Input: dimensioned drawing with shaded views. Units: mm. Origin: part minimum x, y, z. A direction names the side the tool comes from. Round coordinates to 2 decimals unless told otherwise and drop trailing zeros. Write each loop counter-clockwise with the first axis right and the second up, starting at its lowest first coordinate (ties: lowest second). Pieces come first, ordered by that corner, then holes. Notation, with made-up numbers: M -13,34.25 L 37,34.25 A11 cw 37,53.25 Z; hole C 48,80.25 d2. An arc over 180 degrees is marked long. Answer in a Markdown table with one row per item. Add a question column.
Item 1: Material intervals for probe 1 along Y at (x, z) = (6.35, 1.75) (1 decimal); probe 2 along Z at (x, y) = (8, 80); probe 3 along Y at (x, z) = (6.25, 0.5), sorted ascending.
Item 2: Set-up query: the marked faces 1, 2 and 3. Return all of +Z, -Z, +X, -X, +Y, -Y with unobstructed straight access to the full face (end or side cutting, diameter ignored); none if empty.
Item 3: Cut plane A-A on x = 6.35. Give the number of separate pieces and of enclosed holes in the cut face, and give its area (3 significant figures).
Item 4: Cut plane D-D on x = 1. Return loops of the section in (y, z).
Item 5: Contact query for flat-ended pins moving along their axis: pin 1 (1.5 mm diameter, centred on x = 1.5, y = 91.5, fed in from +Z); pin 2 (0.8 mm diameter, centred on x = 7.5, z = 5.5, fed in from +Y); pin 3 (3 mm diameter, centred on x = 6.35, y = 98.425, fed in from -Z); pin 4 (4 mm diameter, centred on x = 8.5, y = 18, fed in from -Z). Output: stop coordinate, or through.
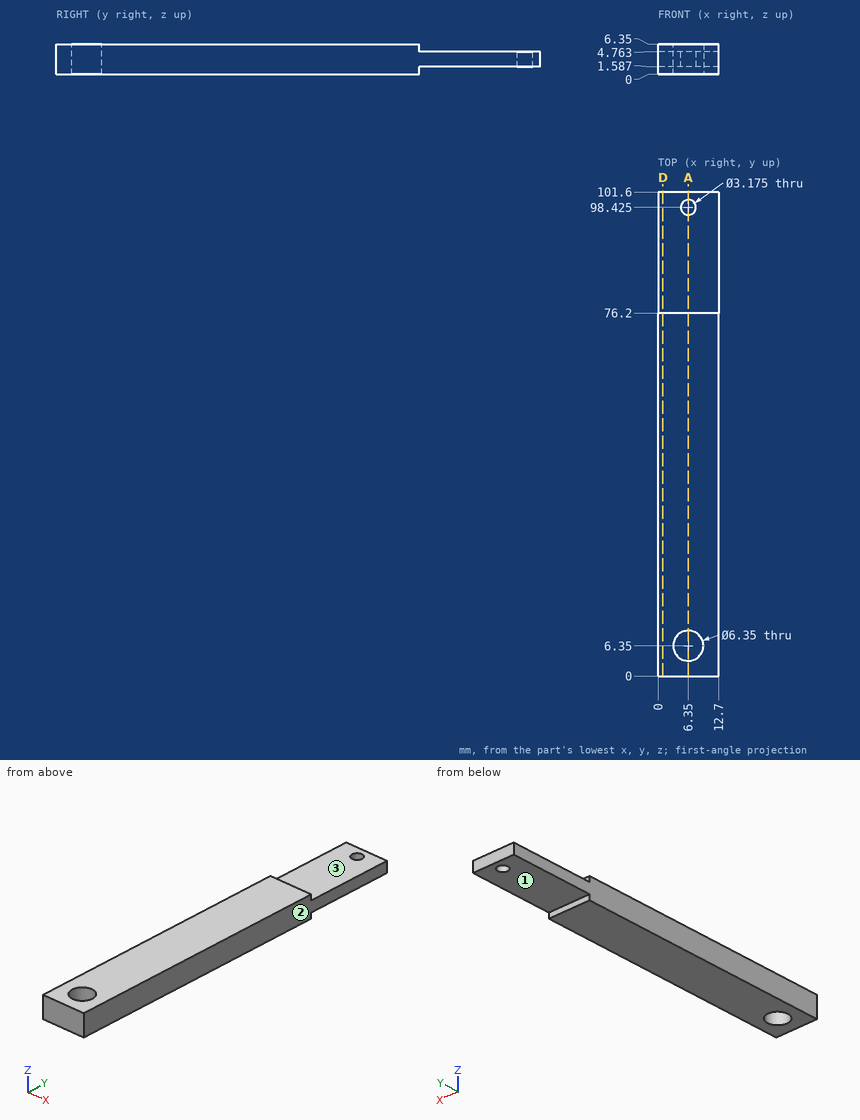
Results below:
| question | item | result |
|---|---|---|
| 1 | probe 1 | 0 to 3.2, 9.5 to 96.8, 100 to 101.6 |
| 1 | probe 2 | 1.59 to 4.76 |
| 1 | probe 3 | 0 to 3.18, 9.52 to 76.2 |
| 2 | face 1 | -Z, +X, -X, +Y |
| 2 | face 2 | +Z, -Z, +X, +Y, -Y |
| 2 | face 3 | +Z, +X, -X, +Y |
| 3 | separate pieces | 3 |
| 3 | enclosed holes | 0 |
| 3 | area | 514 mm2 |
| 4 | outline | M 0,0 L 76.2,0 L 76.2,1.59 L 101.6,1.59 L 101.6,4.76 L 76.2,4.76 L 76.2,6.35 L 0,6.35 Z |
| 5 | pin 1 | z = 4.76 |
| 5 | pin 2 | y = 76.2 |
| 5 | pin 3 | through |
| 5 | pin 4 | z = 0 |
